Verification items for this drawing (mm, ordinates from the low corner). A direction names the side the tool comes from. Round coordinates to 2 decimals unless told otherwise and drop trailing zeros. Order: outer loops, then holes, each group sorted by start corner. A loop starts at its lowest first (then second) coordinate and runs counter-clockwise, first axis right, second up. Notation, with made-up numbers: (19, 3.5) -> (63, 3.5) arc R17 ccw to (63, 30.5) -> close; hole circle Ø8 at (76.25, 75). An arc over 180 degrees is marked (long way). Answer in a Markdown table with one row per item.
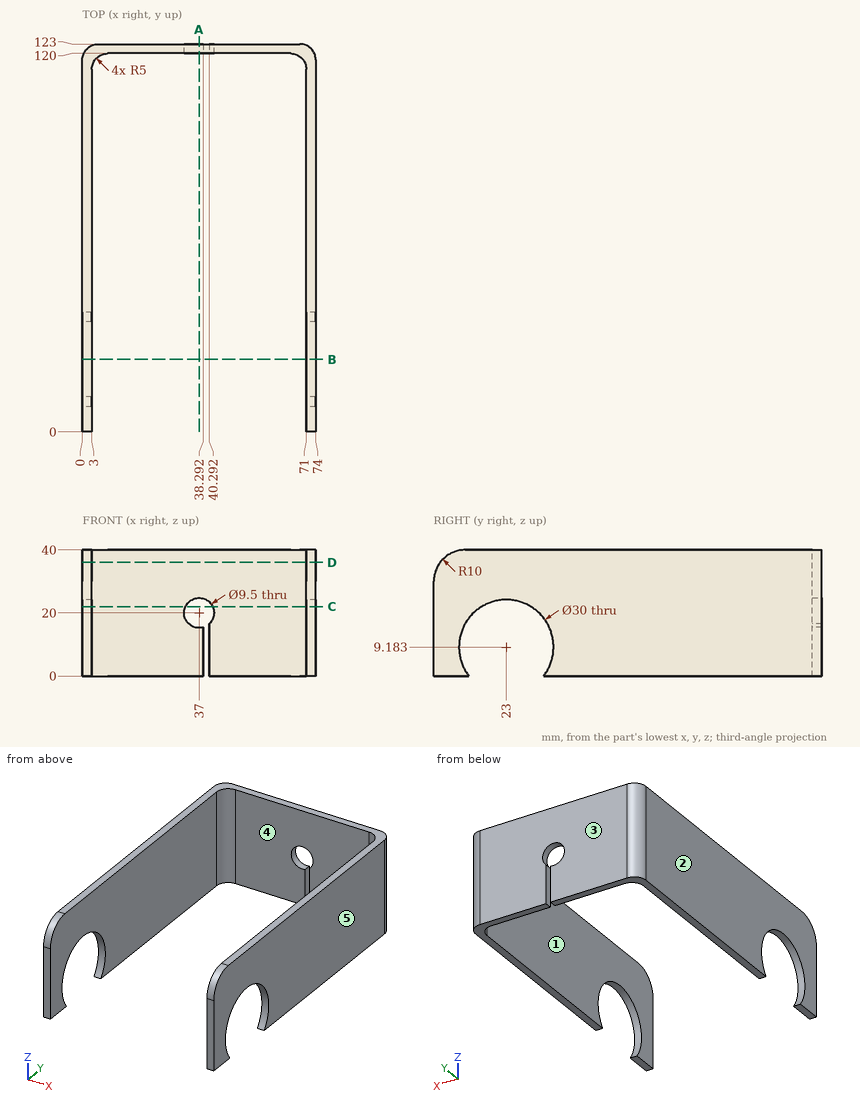
Item 1: Cross-section at C-C (z = 22). Record the boundary of the cut face in (x, y).
Result sheet:
| item | result |
|---|---|
| outline | (0, 0) -> (3, 0) -> (3, 15.21) -> (0, 15.21) -> close; (0, 30.79) -> (3, 30.79) -> (3, 115) arc R5 cw to (8, 120) -> (32.69, 120) -> (32.69, 123) -> (5, 123) arc R5 ccw to (0, 118) -> close; (41.31, 120) -> (66, 120) arc R5 cw to (71, 115) -> (71, 30.79) -> (74, 30.79) -> (74, 118) arc R5 ccw to (69, 123) -> (41.31, 123) -> close; (71, 0) -> (74, 0) -> (74, 15.21) -> (71, 15.21) -> close |
Item 2: Depth check by flat-ended pin: P1, Ø20, axis at x = 29, z = 13.5, coming from the -Y side; P2, Ø1.5, axis at y = 121.5, z = 8, coming from the -X side (1 decimal); P3, Ø0.9, axis at y = 121, z = 9, coming from the +X side. Enter the tip coordinate at first touch or a pass-through.
Result sheet:
| item | result |
|---|---|
| P1 | stops at y = 120 |
| P2 | stops at x = 0.8 |
| P3 | stops at x = 73.3 |
Item 3: Set-up check for the marked faces 4 and 5: record each of +Z, -Z, +X, -X, +Y, -Y from which the full face is reachable in a straight line by a thin tool's end or side.
Result sheet:
| item | result |
|---|---|
| face 4 | +Z, -Z, -Y |
| face 5 | +Z, -Z, +X, +Y, -Y |
Item 4: Cross-section at A-A (x = 37). Record the boundary of the cut face in (y, z).
Result sheet:
| item | result |
|---|---|
| outline | (120, 0) -> (123, 0) -> (123, 15.25) -> (120, 15.25) -> close; (120, 24.75) -> (123, 24.75) -> (123, 40) -> (120, 40) -> close |
Item 5: Mould release check, pull along X, two halves, no side actions. Record for the marked faces 1, 2 and 3: pulls with the +X half, pulls with the -X half, needs draft (parallel to the pull), parting line crosses it, or undercut.
Result sheet:
| item | result |
|---|---|
| face 1 | undercut |
| face 2 | pulls with the -X half |
| face 3 | needs draft |
Item 6: Scan lines: line 1 (X direction, y = 33.5, z = 35); line 2 (Y direction, x = 37.5, z = 35.5); line 3 (Z direction, x = 37, y = 122.15). Record each from-to range of solid material in increasing order. Write a range as [from, to].
Result sheet:
| item | result |
|---|---|
| line 1 | x = [0, 3], [71, 74] |
| line 2 | y = [120, 123] |
| line 3 | z = [0, 15.25], [24.75, 40] |
Item 7: Cross-section at D-D (z = 36). Record the boundary of the cut face in (x, y).
Result sheet:
| item | result |
|---|---|
| outline | (0, 2) -> (3, 2) -> (3, 115) arc R5 cw to (8, 120) -> (66, 120) arc R5 cw to (71, 115) -> (71, 2) -> (74, 2) -> (74, 118) arc R5 ccw to (69, 123) -> (5, 123) arc R5 ccw to (0, 118) -> close |
Item 8: Cross-section at B-B (y = 23). Record the boundary of the cut face in (x, z).
Result sheet:
| item | result |
|---|---|
| outline | (0, 24.18) -> (3, 24.18) -> (3, 40) -> (0, 40) -> close; (71, 24.18) -> (74, 24.18) -> (74, 40) -> (71, 40) -> close |
